Build history of the part. All positions in model axes, mm. A direction names the side the tool comes from. Give positions to 0.01 mm unless a question says otherwise; leave off trailing zeros. Order: outer loops, then holes, each group sorted by start corner. A loop starts at its lowest first (then second) coordinate and runs counter-clockwise, first axis right, second up. Notation, with made-up numbers: (34.25, 44) - (48.25, 44) arc R15 ccw to (48.25, 64) - close; hole circle Ø8 at (-34, 38.5). An arc over 180 degrees is marked (long way). Answer in a Markdown table with one row per item.
```python
from build123d import *

# Parameters (mm, degrees)
SKETCH1_W           = 9.95
SKETCH1_H           = 11.95
BOSS_EXTRUDE2_DEPTH = 5
BOSS_EXTRUDE4_DEPTH = 27.23
SKETCH3_W           = 29
SKETCH3_H           = 14.7
BOSS_EXTRUDE5_DEPTH = 3
BOSS_EXTRUDE6_DEPTH = 35.6
SKETCH7_W           = 29
SKETCH7_H           = 14.7
BOSS_EXTRUDE7_DEPTH = 5.37
SKETCH8_R           = 3.75
BOSS_EXTRUDE8_DEPTH = 35.6


with BuildPart() as part:
    # Sketch1 → Boss-Extrude2 (new body)
    with BuildSketch(Plane(origin=(0, 0, 0), x_dir=(1, 0, 0), z_dir=(0, 1, 0))):
        with BuildLine():
            Line((35.355339059, -35.355339059), (7.975, -7.975))
            Line((7.975, -7.975), (7.975, 8.975))
            Line((7.975, 8.975), (3.717566722, 8.975))
            Line((3.717566722, 8.975), (19.134171618, 46.193976626))
            ThreePointArc((19.134171618, 46.193976626), (-48.299723588, 12.928136036), (-6.5, -49.575699692))
            Line((-6.5, -49.575699692), (-6.5, -42))
            ThreePointArc((-6.5, -42), (-1.406857491, -35.654075954), (5.891000616, -39.252981299))
            Line((5.891000616, -39.252981299), (10.393160878, -48.907895139))
            ThreePointArc((10.393160878, -48.907895139), (23.856849241, -43.941446771), (35.355339059, -35.355339059))
        make_face()
        Rectangle(SKETCH1_W, SKETCH1_H, mode=Mode.SUBTRACT)
    extrude(amount=BOSS_EXTRUDE2_DEPTH)

    # Sketch2 → Boss-Extrude4 (add)
    with BuildSketch(Plane(origin=(0, 5, 0), x_dir=(1, 0, 0), z_dir=(0, 1, 0))):
        with BuildLine():
            Line((17.15, -61.7), (-5.85, -61.7))
            Line((-5.85, -61.7), (-5.85, -50))
            Line((-5.85, -50), (-6.5, -49.575699692))
            ThreePointArc((-6.5, -49.575699692), (-7.67717135, -49.407095038), (-8.85, -49.21054257))
            Line((-8.85, -49.21054257), (-8.85, -64.7))
            Line((-8.85, -64.7), (20.15, -64.7))
            Line((20.15, -64.7), (20.15, -50))
            Line((20.15, -50), (20.15, -45.759998907))
            ThreePointArc((20.15, -45.759998907), (18.65975815, -46.387643029), (17.15, -46.966770168))
            Line((17.15, -46.966770168), (17.15, -50))
            Line((17.15, -50), (17.15, -61.7))
        make_face()
        with BuildLine():
            ThreePointArc((-8.85, -49.21054257), (-7.67717135, -49.407095038), (-6.5, -49.575699692))
            Line((-6.5, -49.575699692), (-6.5, -42))
            Line((-6.5, -42), (-8.85, -42))
            Line((-8.85, -42), (-8.85, -49.21054257))
        make_face()
        with BuildLine():
            Line((17.15, -42), (17.15, -46.966770168))
            ThreePointArc((17.15, -46.966770168), (18.65975815, -46.387643029), (20.15, -45.759998907))
            Line((20.15, -45.759998907), (20.15, -42))
            Line((20.15, -42), (17.15, -42))
        make_face()
    extrude(amount=BOSS_EXTRUDE4_DEPTH)

    # Sketch3 → Boss-Extrude5 (add)
    with BuildSketch(Plane(origin=(0, 32.23, 0), x_dir=(1, 0, 0), z_dir=(0, 1, 0))):
        with Locations((5.65, -57.35)):
            Rectangle(SKETCH3_W, SKETCH3_H)
    extrude(amount=BOSS_EXTRUDE5_DEPTH)

    # Sketch4 → Boss-Extrude6 (add)
    with BuildSketch(Plane(origin=(0, 5, 0), x_dir=(1, 0, 0), z_dir=(0, 1, 0))):
        with BuildLine():
            Line((0, 16.5), (0, 15))
            ThreePointArc((0, 15), (-15, 0), (0, -15))
            Line((0, -15), (0, -16.5))
            ThreePointArc((0, -16.5), (-16.5, 0), (0, 16.5))
        make_face()
    extrude(amount=BOSS_EXTRUDE6_DEPTH)

    # Sketch7 → Boss-Extrude7 (add)
    with BuildSketch(Plane(origin=(0, 35.23, 0), x_dir=(1, 0, 0), z_dir=(0, 1, 0))):
        with Locations((5.65, -57.35)):
            Rectangle(SKETCH7_W, SKETCH7_H)
    extrude(amount=BOSS_EXTRUDE7_DEPTH)

    # Sketch8 → Boss-Extrude8 (add)
    with BuildSketch(Plane(origin=(0, 5, 0), x_dir=(1, 0, 0), z_dir=(0, 1, 0))):
        with Locations(Location((14.176286342, 44.023804987, 0), (0, 0, 72.150709005))):
            Circle(SKETCH8_R)
        with Locations(Location((29.944361597, -35.247662455, 0), (0, 0, 45))):
            Circle(SKETCH8_R)
        with Locations(Location((-46.25, 0, 0), (0, 0, 179.999564815))):
            Circle(SKETCH8_R)
    extrude(amount=BOSS_EXTRUDE8_DEPTH)


solid = part.part
```
1. Cut at C-C on z = -12. Write the cut outline in (x, y).
Check result:
| item | result |
|---|---|
| outline | (-48.54, 0) - (4.97, 0) - (4.97, 5) - (-9, 5) - (-9, 40.6) - (-11.32, 40.6) - (-11.32, 5) - (-48.54, 5) - close |
2. Drop flat-ended pins along their axis: P1, Ø3.5, axis at x = 5.5, y = 2, coming from the -Z side; P2, Ø1.5, axis at y = 16.5, z = 6.5, coming from the +X side; P3, Ø4, axis at x = 2.5, y = 2.5, coming from the +Z side. Give the stop position or say it passes through.
Check result:
| item | result |
|---|---|
| P1 | stops at z = -49.86 |
| P2 | stops at x = -13.13 |
| P3 | stops at z = 37.31 |
3. Cut at B-B on x = -12.5. Write the cut outline in (y, z), and give its area (3 significant figures).
Check result:
| item | result |
|---|---|
| outline | (0, -48.41) - (5, -48.41) - (5, -10.77) - (40.6, -10.77) - (40.6, -8.29) - (5, -8.29) - (5, 8.29) - (40.6, 8.29) - (40.6, 10.77) - (5, 10.77) - (5, 48.41) - (0, 48.41) - close |
| area | 661 mm² |
4. Two-plate mould, pull along X, no slides. Class faces 1 (the face through (-6.5, 16, 46)), 2 (the face through (29.454, 22.551, 38.965)), 3 (the face through (19, 32.23, 46)): +X half, -X half, draft (parallel to the pull), parting line (faces both ways), or undercut.
Check result:
| item | result |
|---|---|
| face 1 | undercut |
| face 2 | parting line |
| face 3 | draft |
5. Probe line 1 (X direction, y = 14, z = 47.5); line 2 (Y direction, x = 12.5, z = 27); line 3 (Z direction, x = 7.5, y = 13). List the from-to ranges inside material, lowest first.
Check result:
| item | result |
|---|---|
| line 1 | x = -8.85 to -6.5, 17.15 to 20.15 |
| line 2 | y = 0 to 5 |
| line 3 | z = 61.7 to 64.7 |
6. Cut at D-D on x = -46.25. Write the cut outline in (y, z).
Check result:
| item | result |
|---|---|
| outline | (0, -19) - (5, -19) - (5, -3.75) - (40.6, -3.75) - (40.6, 3.75) - (5, 3.75) - (5, 19) - (0, 19) - close |
7. Cut at A-A on y = 27. Write the cut outline in (x, z).
Check result:
| item | result |
|---|---|
| outline | circle Ø7.5 at (-46.25, 0); (-8.85, 42) - (-6.5, 42) - (-6.5, 49.58) - (-5.85, 50) - (-5.85, 61.7) - (17.15, 61.7) - (17.15, 42) - (20.15, 42) - (20.15, 64.7) - (-8.85, 64.7) - close; (0, -16.5) - (0, -15) arc R15 cw to (0, 15) - (0, 16.5) arc R16.5 ccw to start; circle Ø7.5 at (14.18, -44.02); circle Ø7.5 at (29.94, 35.25) |
8. Which spindle directions (+Z, -Z, +X, -X, +Y, -Y) get a long thin tool onto all of the face, cutting with end or side? Do faces 4 (the face through (-8.85, 23, 54)), 5 (the face through (0, 2, -5.975)), 6 (the face through (7.975, 2, 0)), 7 (the face through (19, 18, 42)). Say none if no direction does.
Check result:
| item | result |
|---|---|
| face 4 | +Z, -X, +Y |
| face 5 | +Y, -Y |
| face 6 | +X, +Y, -Y |
| face 7 | +X, -X, +Y |
